```python
from build123d import *

# Parameters (mm, degrees)
F1_DEPTH = 127
F2_R     = 2
F3_R     = 4
F4_R     = 6
F5_R     = 4
F6_R     = 1.625
F7_DEPTH = 2
F8_R     = 1.75
F9_DEPTH = 2


with BuildPart() as f1:
    # F0 (on Right) → F1 (new body, symmetric)
    with BuildSketch(Plane.YZ):
        Polygon((-82, 0), (0, 0), (0, 320), (-2, 320), (-2, 2), (-82, 2), align=None)
    extrude(amount=F1_DEPTH, both=True)

    # F2
    f2_edges = [f1.edges().sort_by_distance(p)[0] for p in [
        (0, -2, 2),
    ]]
    fillet(f2_edges, radius=F2_R)

    # F3
    f3_edges = [f1.edges().sort_by_distance(p)[0] for p in [
        (0, 0, 0),
    ]]
    fillet(f3_edges, radius=F3_R)

    # F4
    f4_edges = [f1.edges().sort_by_distance(p)[0] for p in [
        (127, -1, 320),
        (-127, -1, 320),
    ]]
    fillet(f4_edges, radius=F4_R)

    # F5
    f5_edges = [f1.edges().sort_by_distance(p)[0] for p in [
        (127, -82, 1),
        (-127, -82, 1),
    ]]
    fillet(f5_edges, radius=F5_R)

    # F6 (on face) → F7 (cut, through all)
    with BuildSketch(Plane(origin=(0, 0, 0), x_dir=(1, 0, 0), z_dir=(0, 0, -1))):
        with Locations((95, 41)):
            Circle(F6_R)
        with Locations((-95, 41)):
            Circle(F6_R)
    extrude(amount=-F7_DEPTH, mode=Mode.SUBTRACT)

    # F8 (on face) → F9 (cut, through all)
    with BuildSketch(Plane(origin=(0, 0, 0), x_dir=(-1, 0, 0), z_dir=(0, 1, 0))):
        with Locations((117.5, 202)):
            Circle(F8_R)
        with Locations((-117.5, 202)):
            Circle(F8_R)
        with Locations((117.5, 62.6)):
            Circle(F8_R)
        with Locations((-117.5, 62.6)):
            Circle(F8_R)
    extrude(amount=-F9_DEPTH, mode=Mode.SUBTRACT)


solid = f1.part
```
Check sheet for the modelled part. Datum: model origin and axes. Units: mm. A direction names the side the tool comes from. Give positions to 0.01 mm unless a question says otherwise; leave off trailing zeros. Write each loop counter-clockwise with the first axis right and the second up, starting at its lowest first coordinate (ties: lowest second). Pieces come first, ordered by that corner, then holes. Notation, with made-up numbers: (65.5, -11.75) - (91.5, -11.75) arc R29 ccw to (91.5, 9.25) - close; hole circle Ø7 at (69.5, 82). An arc over 180 degrees is marked (long way). Answer as a JSON object with one key per item and string values. Group by question number.
1) Sectioned sample at C-C (y = -18.5). Record the cut outline in (x, z).
2) Depth check by flat-ended pin: P1, Ø3, axis at x = -117.5, z = 202, coming from the -Y side; P2, Ø12, axis at x = -54.5, z = 245, coming from the -Y side; P3, Ø3, axis at x = 55, y = -15.5, coming from the +Z side. Enter the tip coordinate at first touch or a pass-through.
3) Sectioned sample at B-B (z = 264). Record the cut outline in (x, y), then the cut area to 3 significant figures.
4) Access from +Z, -Z, +X, -X, +Y, -Y to the whole of each face (thin tool, end or side, straight path). Record for faces 1 (the face through (127, -1.6, 157.7)), 2 (the face through (2, -2, 164)).
5) Thickness scan on probe 1 along X at (y, z) = (-41, 1.1) (3 decimals); probe 2 along Z at (x, y) = (-117.5, -0.5); probe 3 along Z at (x, y) = (117.5, -0.7). Record the ranges inside material, lowest first. Write a range as from..to.
6) Sectioned sample at A-A (x = 38). Record the cut outline in (y, z), then the cut area to 3 significant figures.
Geometry results:
{
 "1": {"outline": "(-127, 0) - (127, 0) - (127, 2) - (-127, 2) - close"},
 "2": {"P1": "passes through", "P2": "stops at y = -2", "P3": "stops at z = 2"},
 "3": {"outline": "(-127, -2) - (127, -2) - (127, 0) - (-127, 0) - close", "area": "508 mm^2"},
 "4": {"face 1": "+Z, -Z, +X, +Y, -Y", "face 2": "+Z, +X, -X, -Y"},
 "5": {"probe 1": "x = -127..-96.625, -93.375..93.375, 96.625..127", "probe 2": "z = 2.06..60.85, 64.35..200.25, 203.75..320", "probe 3": "z = 1.74..60.85, 64.35..200.25, 203.75..320"},
 "6": {"outline": "(-82, 0) - (-4, 0) arc R4 ccw to (0, 4) - (0, 320) - (-2, 320) - (-2, 4) arc R2 cw to (-4, 2) - (-82, 2) - close", "area": "797 mm^2"}
}
